```python
from build123d import *

# Parameters (mm, degrees)
SKETCH1_W                      = 60.325
SKETCH1_H                      = 19.05
BOSS_EXTRUDE1_DEPTH            = 38.1
SKETCH2_R                      = 13.335
CUT_EXTRUDE1_DEPTH             = 20.05
CBORE_FOR_M4_SHCS1_D           = 4.5
CBORE_FOR_M4_SHCS1_CBORE_D     = 8
CBORE_FOR_M4_SHCS1_CBORE_DEPTH = 4
FILLET1_R                      = 2


with BuildPart() as part:
    # Sketch1 → Boss-Extrude1 (new body)
    with BuildSketch(Plane(origin=(0, 0, 0), x_dir=(1, 0, 0), z_dir=(0, 1, 0))):
        Rectangle(SKETCH1_W, SKETCH1_H)
    extrude(amount=BOSS_EXTRUDE1_DEPTH)

    # Sketch2 → Cut-Extrude1 (cut, through all)
    with BuildSketch(Plane.XY.offset(9.525)):
        with Locations((0, 19.05)):
            Circle(SKETCH2_R)
    extrude(amount=-CUT_EXTRUDE1_DEPTH, mode=Mode.SUBTRACT)

    # CBORE for M4 SHCS1 (through all)
    with Locations(Plane(origin=(0, 38.1, 0), x_dir=(1, 0, 0), z_dir=(0, 1, 0))):
        with Locations((-20.6375, 0), (20.6375, 0)):
            CounterBoreHole(CBORE_FOR_M4_SHCS1_D / 2, CBORE_FOR_M4_SHCS1_CBORE_D / 2, CBORE_FOR_M4_SHCS1_CBORE_DEPTH)

    # Fillet1
    fillet1_edges = [part.edges().sort_by_distance(p)[0] for p in [
        (-30.1625, 38.1, 0),
        (30.1625, 38.1, 0),
    ]]
    fillet(fillet1_edges, radius=FILLET1_R)


solid = part.part
```
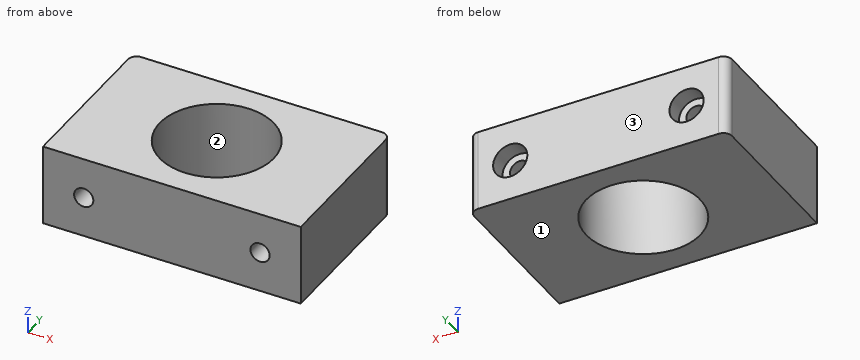
Geometry: final body of the model. Coordinates: model frame, mm. Face numbers are marked on the shaded views. Give positions to 0.01 mm unless a question says otherwise; leave off trailing zeros. Write each loop counter-clockwise with the first axis right and the second up, starting at its lowest first coordinate (ties: lowest second). Pieces come first, ordered by that corner, then holes.
1. Draft query along Y for the marked faces 1, 2 and 3. Return one class per face: released by +Y, released by -Y, zero draft, split by the parting line, or undercut.
2. Section query A-A, the plane y = 19.05. Count the separate pieces of the cut face and the enclosed holes in it, then the cut area to 3 significant figures.
3. Pin query (flat end, axial travel): P1, Ø5, axis at x = -20.64, z = 0, coming from the +Y side. Return the tip coordinate at first contact, or that it passes through.
4. Section query C-C, the plane x = 0. Return loops of the section in (y, z) (3 decimals), then the cut area to 3 significant figures.
5. Line query: probe 1 along X at (y, z) = (10, 1.75); probe 2 along X at (y, z) = (9.5, -0.75); probe 3 along X at (y, z) = (17.5, -8.25). Output: solid intervals per line, ascending.
Computed:
1. face 1: zero draft
1. face 2: undercut
1. face 3: released by +Y
2. separate pieces: 2
2. enclosed holes: 2
2. area: 609 mm2
3. P1: stops at y = 34.1
4. outline: (0, -9.525) - (5.715, -9.525) - (5.715, 9.525) - (0, 9.525) - close; (32.385, -9.525) - (38.1, -9.525) - (38.1, 9.525) - (32.385, 9.525) - close
4. area: 218 mm2
5. probe 1: x = -30.16 to -22.05, -19.22 to -9.79, 9.79 to 19.22, 22.05 to 30.16
5. probe 2: x = -30.16 to -22.76, -18.52 to -9.31, 9.31 to 18.52, 22.76 to 30.16
5. probe 3: x = -30.16 to -13.24, 13.24 to 30.16
